Can you work these out from the drawing? Everything is in mm from the part's minimum corner. Coordinates: 2 decimals unless noted, no trailing zeros. Order: outer loops, then holes, each group sorted by start corner. A loop starts at its lowest first (then second) coordinate and runs counter-clockwise, first axis right, second up. Notation, with made-up numbers: (-18, 80) - (16, 80) arc R9 cw to (16, 93) - close; hole circle Ø3 at (-14, 86.25). An arc over 180 degrees is marked (long way). Use CSV: the item, a comma, the result in double quotes. Start each with the question number.
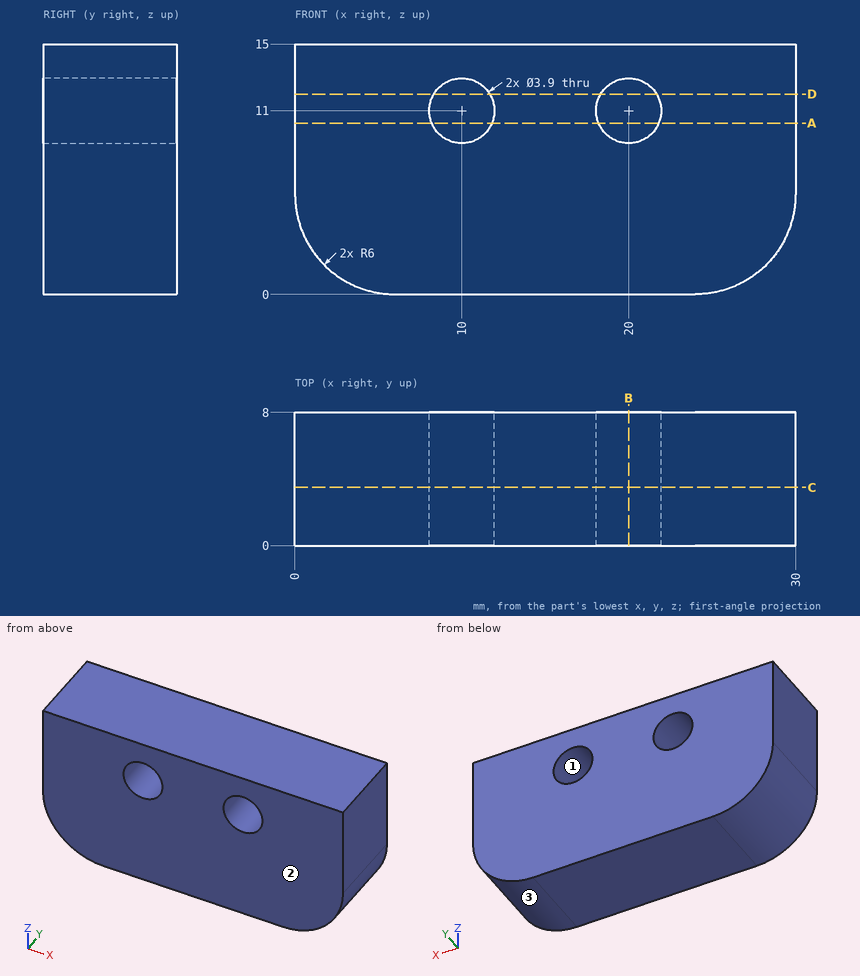
Item 1: Suppose I cut it at D-D on z = 12. Write out the boundary of the cut face in (x, y), then the cut area to 3 significant figures.
Item 2: Please list where these lines run through material, in increasing order: line 1 along X through (y, z) = (2, 11); line 2 along X through (y, z) = (4.75, 12); line 3 along X through (y, z) = (1.5, 2). Write a range as from..to.
Item 3: Suppose I cut it at A-A on z = 10.25. Write out the boundary of the cut face in (x, y).
Item 4: Suppose I cut it at C-C on y = 3.5. Write out the boundary of the cut face in (x, z), then the cut area to 3 significant figures.
Item 5: Suppose I cut it at B-B on x = 20. Write out the boundary of the cut face in (y, z).
Item 6: We'd pull the mould along Z, two halves only. Please class the marked faces 1, 2 and 3: released by +Z, released by -Z, zero draft, split by the parting line, or undercut.
Item 7: For pin 1 Ø3.5 at (x, z) = (10, 11) entering from +Y; pin 2 Ø1 at (x, y) = (4, 3) entering from -Z, each with a flat end and sliding along its axis, tell me the tip position at first contact or that it passes through.
Here are the results:
1,outline,"(0, 0) - (8.33, 0) - (8.33, 8) - (0, 8) - close; (11.67, 0) - (18.33, 0) - (18.33, 8) - (11.67, 8) - close; (21.67, 0) - (30, 0) - (30, 8) - (21.67, 8) - close"
1,area,"186 mm^2"
2,line 1,"0..8.05, 11.95..18.05, 21.95..30"
2,line 2,"0..8.33, 11.67..18.33, 21.67..30"
2,line 3,"1.53..28.47"
3,outline,"(0, 0) - (8.2, 0) - (8.2, 8) - (0, 8) - close; (11.8, 0) - (18.2, 0) - (18.2, 8) - (11.8, 8) - close; (21.8, 0) - (30, 0) - (30, 8) - (21.8, 8) - close"
4,outline,"(0, 6) arc R6 ccw to (6, 0) - (24, 0) arc R6 ccw to (30, 6) - (30, 15) - (0, 15) - close; hole circle Ø3.9 at (10, 11); hole circle Ø3.9 at (20, 11)"
4,area,"411 mm^2"
5,outline,"(0, 0) - (8, 0) - (8, 9.05) - (0, 9.05) - close; (0, 12.95) - (8, 12.95) - (8, 15) - (0, 15) - close"
6,face 1,"undercut"
6,face 2,"zero draft"
6,face 3,"released by -Z"
7,pin 1,"through"
7,pin 2,"z = 0.19"
